from build123d import *

# Parameters (mm, degrees)
F1_DEPTH = 2
F2_R     = 0.5


with BuildPart() as f1:
    # F0 (on Top) → F1 (new body)
    with BuildSketch(Plane.XY):
        with BuildLine():
            ThreePointArc((-42.5555160352, 38.8332652748), (-47.2791269422, 44.0832652748), (-52.0027378491, 38.8332652748))
            Line((-52.0027378491, 38.8332652748), (-42.5555160352, 38.8332652748))
        make_face()
        with BuildLine():
            ThreePointArc((-51.5291269422, 39.3332652748), (-47.2791269422, 43.5832652748), (-43.0291269422, 39.3332652748))
            Line((-43.0291269422, 39.3332652748), (-51.5291269422, 39.3332652748))
        make_face(mode=Mode.SUBTRACT)
    extrude(amount=F1_DEPTH)

    # F2
    f2_edges = [f1.edges().sort_by_distance(p)[0] for p in [
        (-52.002738, 38.833265, 1),
        (-42.555516, 38.833265, 1),
    ]]
    fillet(f2_edges, radius=F2_R)


solid = f1.part
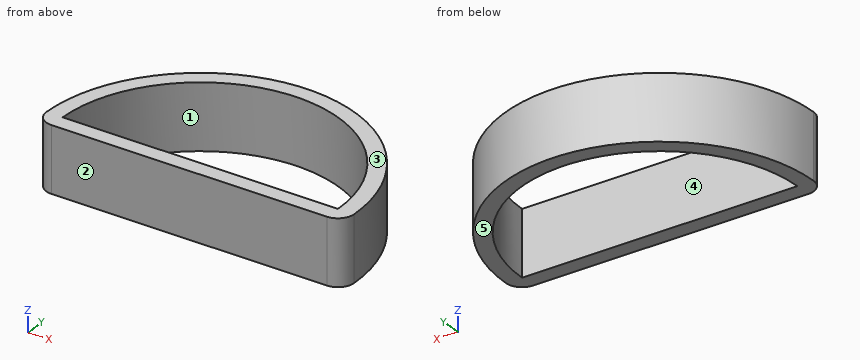
The model under review builds one solid part; all positions refer to its coordinate system, in mm. Face numbers are marked on the shaded views. A direction names the side the tool comes from. Round coordinates to 2 decimals unless told otherwise and drop trailing zeros. Write each loop counter-clockwise with the first axis right and the second up, starting at its lowest first coordinate (ties: lowest second). Pieces come first, ordered by that corner, then holes. Notation, with made-up numbers: M 0,-29 L 13,-29 A29 cw 13,2 Z; hole C 33,5 d9. An arc over 180 degrees is marked long. Answer as CSV lines item,"result". Start each with the question number.
Q1. Consider section C-C, the plane y = 40. Give the boundary of the cut face in (x, z), then the cut area to 3 significant figures.
Q2. The part is to be moulded in two halves that separate along Z. For the marked faces 3, 4 and 5, say which applies: +Z half, -Z half, draft (parallel to the pull), parting line (faces both ways), or undercut.
Q3. Consider section A-A, the plane x = -48.5. Give the boundary of the cut face in (y, z).
Q4. Consider section B-B, the plane z = 1.7. Give the boundary of the cut face in (x, y), then the cut area to 3 significant figures.
Q5. Tool access review of the marked faces 1 and 2: name each direction out of +Z, -Z, +X, -X, +Y, -Y from which nothing blocks a thin tool from reaching the whole face with its end or side.
Q6. Wall thickness on line 1 along X through (y, z) = (39.4, 1.1); line 2 along Y through (x, z) = (-47, 1.6); line 3 along Y through (x, z) = (-46, 0.7): over which ranges is each line inside the solid? List them lowest first.
Q7. Clearance check with flat-ended pins moving along their axes: P1, Ø1.5, axis at x = -47, y = 42.5, coming from the -Z side; P2, Ø1, axis at x = -46.5, z = 1, coming from the +Y side. State where each tip first meets the part, or that it passes through.
Result set:
1,outline,"M -51.98,0 L -51.48,0 L -51.48,2 L -51.98,2 Z; M -43.08,0 L -42.58,0 L -42.58,2 L -43.08,2 Z"
1,area,"2.02 mm²"
2,face 3,"+Z half"
2,face 4,"draft"
2,face 5,"-Z half"
3,outline,"M 38.83,0 L 39.33,0 L 39.33,2 L 38.83,2 Z; M 43.4,0 L 43.92,0 L 43.92,2 L 43.4,2 Z"
4,outline,"M -52.03,39.33 A0.5 ccw -51.53,38.83 L -43.03,38.83 A0.5 ccw -42.53,39.33 A4.75 ccw Z; hole M -51.53,39.33 L -43.03,39.33 A4.25 ccw Z"
4,area,"11.7 mm²"
5,face 1,"+Z, -Z"
5,face 2,"+Z, -Z, +X, -X, -Y"
6,line 1,"x = -52.03 to -51.53, -43.03 to -42.53"
6,line 2,"y = 38.83 to 39.33, 43.57 to 44.08"
6,line 3,"y = 38.83 to 39.33, 43.39 to 43.91"
7,P1,"passes through"
7,P2,"stops at y = 44.08"
